The listing builds one solid part. Answer for the finished solid, in the listing's coordinates (mm). Face numbers are marked on the shaded views. A direction names the side the tool comes from. Coordinates: 2 decimals unless noted, no trailing zeros. Loops run counter-clockwise (first coordinate to the right, second up) from the corner with the lowest first, then second, coordinate; pieces in that order, holes last. Notation, with made-up numbers: M 67.5,-23.5 L 119.5,-23.5 A23 cw 119.5,-4.5 Z; hole C 38,2 d5. An arc over 180 degrees is marked long. Answer as a JSON object with one key per item and string values. Group by question number.
1. A cutting plane is placed at C-C on y = -8.75. Give the vertices of the cut face in (x, z).
2. A cutting plane is placed at A-A on y = -1. Give the vertices of the cut face in (x, z).
3. A cutting plane is placed at B-B on z = 0. Give the vertices of the cut face in (x, y), and give its area (3 significant figures).
4. Straight lines are drawn through the part: L1, parallel to Y at x = -2.75, z = -1; L2, parallel to X at y = -1.5, z = 0.5; L3, parallel to X at y = -5, z = 1.75. For each, find the intervals that lie inside material, in ascending order.
5. For the marked faces 1, 2 and 3, determine the directions among +Z, -Z, +X, -X, +Y, -Y from which every point of the face is accessible in a straight line to the end or side of a thin tool.
6. Given pin 1 (0.9 mm diameter, centred on x = -0.5, z = 0, fed in from +Y); pin 2 (2 mm diameter, centred on x = -2, z = 2.5, fed in from -Y); pin 3 (3 mm diameter, centred on y = -4, z = 2, fed in from +X), each flat-ended and moving along its own axis, determine where each tip first touches the part or whether it passes through.
7. Determine the mould class of the marked faces 4, 5, 6 and 7 for opening direction X: released by +X, released by -X, zero draft, split by the parting line, or undercut.
from build123d import *

# Parameters (mm, degrees)
CORTAR_EXTRUIR1_DEPTH = 3
CHAFL_N1_SIZE         = 0.5
REDONDEO1_R           = 0.5


with BuildPart() as part:
    # Croquis1 → Revolución1 (revolve)
    with BuildSketch(Plane.XY):
        Polygon((0, 0), (3.5, 0), (3.5, -4), (2, -4), (2, -10), (0, -10), align=None)
    revolve(axis=Axis((0, 0, 0), (0, -1, 0)))

    # Croquis2 → Cortar-Extruir1 (cut)
    with BuildSketch(Plane(origin=(0, 0, 0), x_dir=(1, 0, 0), z_dir=(0, 1, 0))):
        Polygon((1.5, 0.866025404), (0, 1.732050808), (-1.5, 0.866025404), (-1.5, -0.866025404), (0, -1.732050808), (1.5, -0.866025404), align=None)
    extrude(amount=-CORTAR_EXTRUIR1_DEPTH, mode=Mode.SUBTRACT)

    # Chaflán1
    chafl_n1_edges = [part.edges().sort_by_distance(p)[0] for p in [
        (-2, -10, 0),
    ]]
    chamfer(chafl_n1_edges, length=CHAFL_N1_SIZE)

    # Redondeo1
    redondeo1_edges = [part.edges().sort_by_distance(p)[0] for p in [
        (-3.5, 0, 0),
    ]]
    fillet(redondeo1_edges, radius=REDONDEO1_R)


solid = part.part
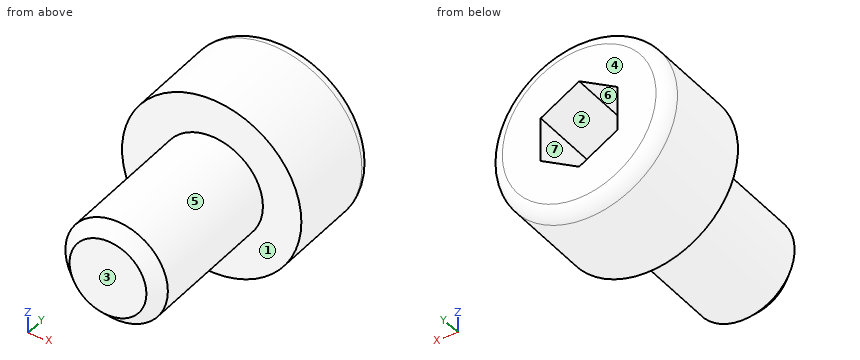
From the geometry:
{
 "1": {"outline": "C 0,0 d4"},
 "2": {"outline": "C 0,0 d7; hole M -1.5,-0.87 L 0,-1.73 L 1.5,-0.87 L 1.5,0.87 L 0,1.73 L -1.5,0.87 Z"},
 "3": {"outline": "M -3.5,-4 L -2,-4 L -2,-9.5 L -1.5,-10 L 1.5,-10 L 2,-9.5 L 2,-4 L 3.5,-4 L 3.5,-0.5 A0.5 ccw 3,0 L 1.5,0 L 1.5,-3 L -1.5,-3 L -1.5,0 L -3,0 A0.5 ccw -3.5,-0.5 Z", "area": "42.6 mm²"},
 "4": {"L1": "y = -4 to 0", "L2": "x = -3.46 to -1.5, 1.5 to 3.46", "L3": "x = -0.97 to 0.97"},
 "5": {"face 1": "-Y", "face 2": "+Y", "face 3": "+Z, -Z, +X, -X, -Y"},
 "6": {"pin 1": "stops at y = -3", "pin 2": "stops at y = -4", "pin 3": "stops at x = 3.46"},
 "7": {"face 4": "zero draft", "face 5": "split by the parting line", "face 6": "undercut", "face 7": "undercut"}
}
